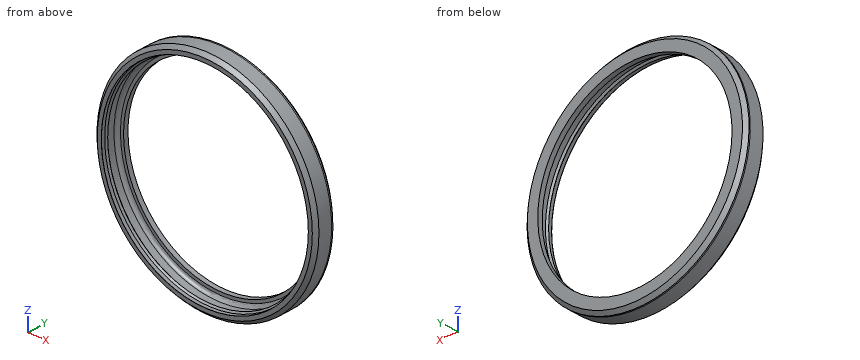
from build123d import *
from build123d.topology import SkipClean

# Parameters (mm, degrees)
SKETCH_1_R          = 32
EXTRUDE_1_DEPTH     = 2.4
SKETCH_3_R          = 28
CUT_EXTRUDE_1_DEPTH = 10
SKETCH_4_R          = 32
CUT_EXTRUDE_2_DEPTH = 1
CHAMFER_1_SIZE      = 1
CHAMFER_2_SIZE      = 1


with BuildPart() as part:
    # Sketch 1 → Extrude 1 (new body)
    with BuildSketch(Plane(origin=(0, 0, 0), x_dir=(1, 0, 0), z_dir=(0, 1, 0))):
        with Locations(Location((0, 0, 0), (0, 0, 270))):
            Circle(SKETCH_1_R)
    extrude(amount=EXTRUDE_1_DEPTH)

    # Sketch 2 → Revolve 1 (revolve)
    with SkipClean():  # the faces are left unmerged after this step: merging them gives an invalid solid
        with BuildSketch(Plane.XY):
            with BuildLine():
                Line((32, 0), (28.897619048, 0))
                ThreePointArc((28.897619048, 0), (29.573809524, -0.30952381), (29.85, -1))
                Line((29.85, -1), (29.85, -3.020710678))
                Line((29.85, -3.020710678), (29.370710678, -3.5))
                Line((29.370710678, -3.5), (29.828219647, -3.957508969))
                Line((29.828219647, -3.957508969), (29.85, -4.95))
                Line((29.85, -4.95), (29.85, -5))
                Line((29.85, -5), (31, -5))
                Line((31, -5), (32, -5))
                Line((32, -5), (32, 0))
            make_face()
        revolve(axis=Axis((0, -25, 0), (0, 1, 0)))
    add(part.part.scale(1), mode=Mode.REPLACE)  # the faces are merged on a copy

    # Sketch 3 → Cut-Extrude 1 (cut)
    with BuildSketch(Plane(origin=(0, 2.4, 0), x_dir=(1, 0, 0), z_dir=(0, 1, 0))):
        with Locations(Location((0, 0, 0), (0, 0, 270))):
            Circle(SKETCH_3_R)
    extrude(amount=-CUT_EXTRUDE_1_DEPTH, mode=Mode.SUBTRACT)

    # Sketch 4 → Cut-Extrude 2 (cut)
    with BuildSketch(Plane(origin=(0, 2.4, 0), x_dir=(1, 0, 0), z_dir=(0, 1, 0))):
        Circle(SKETCH_4_R)
    extrude(amount=-CUT_EXTRUDE_2_DEPTH, mode=Mode.SUBTRACT)

    # Chamfer 1
    chamfer_1_edges = [part.edges().sort_by_distance(p)[0] for p in [
        (-32, -5, 0),
    ]]
    chamfer(chamfer_1_edges, length=CHAMFER_1_SIZE)

    # Chamfer 2
    chamfer_2_edges = [part.edges().sort_by_distance(p)[0] for p in [
        (0, 1.4, -32),
    ]]
    chamfer(chamfer_2_edges, length=CHAMFER_2_SIZE)


solid = part.part
Design review of the part built by this model. Coordinates are the model's own, in mm. Round coordinates to 2 decimals unless told otherwise and drop trailing zeros. Write each loop counter-clockwise with the first axis right and the second up, starting at its lowest first coordinate (ties: lowest second). Pieces come first, ordered by that corner, then holes.
Item 1: Consider section C-C on z = 0. Give the boundary of the cut face in (x, y), and give its area (3 significant figures).
Item 2: Consider section A-A on x = 0. Give the boundary of the cut face in (y, z), and give its area (3 significant figures).
Item 3: For pin 1 Ø3 at (x, y) = (19.5, -3.5) entering from +Z; pin 2 Ø1.5 at (y, z) = (-4, -1.5) entering from -X; pin 3 Ø2 at (x, y) = (6, -4) entering from +Z, all flat-tipped, find the tip position at first contact; note any pin that passes through.
Item 4: Wall thickness on L1, parallel to X at y = -2, z = 0; L2, parallel to Z at x = -16, y = -4.25: over which ranges is each line inside the solid? List them lowest first.
Item 5: Consider section B-B on y = -2.25. Give the boundary of the cut face in (x, z).
Check values:
1. outline: (-32, -4) - (-31, -5) - (-29.85, -5) - (-29.85, -4.95) - (-29.83, -3.96) - (-29.37, -3.5) - (-29.85, -3.02) - (-29.85, -1) arc R1 cw to (-28.9, 0) - (-28, 0) - (-28, 1.4) - (-31, 1.4) - (-32, 0.4) - close; (28, 0) - (28.9, 0) arc R1 cw to (29.85, -1) - (29.85, -3.02) - (29.37, -3.5) - (29.83, -3.96) - (29.85, -4.95) - (29.85, -5) - (31, -5) - (32, -4) - (32, 0.4) - (31, 1.4) - (28, 1.4) - close
1. area: 31.6 mm2
2. outline: (-5, -31) - (-4, -32) - (0.4, -32) - (1.4, -31) - (1.4, -28) - (0, -28) - (0, -28.9) arc R1 cw to (-1, -29.85) - (-3.02, -29.85) - (-3.5, -29.37) - (-3.96, -29.83) - (-4.95, -29.85) - (-5, -29.85) - close; (-5, 29.85) - (-4.95, 29.85) - (-3.96, 29.83) - (-3.5, 29.37) - (-3.02, 29.85) - (-1, 29.85) arc R1 cw to (0, 28.9) - (0, 28) - (1.4, 28) - (1.4, 31) - (0.4, 32) - (-4, 32) - (-5, 31) - close
2. area: 31.6 mm2
3. pin 1: stops at z = 26.46
3. pin 2: stops at x = -31.99
3. pin 3: stops at z = 31.61
4. L1: x = -32 to -29.85, 29.85 to 32
4. L2: z = -27.42 to -25.18, 25.18 to 27.42
5. outline: circle Ø64 at (0, 0); hole circle Ø59.7 at (0, 0)
